Check sheet for the modelled part. Datum: model origin and axes. Units: mm. Coordinates: 2 decimals unless noted, no trailing zeros. Loops run counter-clockwise (first coordinate to the right, second up) from the corner with the lowest first, then second, coordinate; pieces in that order, holes last. Notation, with made-up numbers: M 71.5,57.25 L 95.5,57.25 A30 ccw 95.5,86.25 Z; hole C 62.25,54 d8. An arc over 180 degrees is marked long. Write each question's results on one line, items separated by ' | '. Start each with the question number.
from build123d import *

# Parameters (mm, degrees)
SKETCH1_R           = 16.1655
BOSS_EXTRUDE1_DEPTH = 13.5
FILLET1_R           = 1
SKETCH2_R           = 12.5
SKETCH2_R_2         = 11
BOSS_EXTRUDE2_DEPTH = 1
FILLET4_R           = 0.707


with BuildPart() as part:
    # Sketch1 → Boss-Extrude1 (new body)
    with BuildSketch(Plane(origin=(0, 0, 0), x_dir=(1, 0, 0), z_dir=(0, 1, 0))):
        Circle(SKETCH1_R)
    extrude(amount=BOSS_EXTRUDE1_DEPTH)

    # Fillet1
    fillet1_edges = [part.edges().sort_by_distance(p)[0] for p in [
        (-16.1655, 0, 0),
        (-16.1655, 13.5, 0),
    ]]
    fillet(fillet1_edges, radius=FILLET1_R)

    # Sketch2 → Boss-Extrude2 (add)
    with BuildSketch(Plane(origin=(0, 13.5, 0), x_dir=(1, 0, 0), z_dir=(0, 1, 0))):
        Circle(SKETCH2_R)
        Circle(SKETCH2_R_2, mode=Mode.SUBTRACT)
    extrude(amount=BOSS_EXTRUDE2_DEPTH)

    # Fillet4
    fillet4_edges = [part.edges().sort_by_distance(p)[0] for p in [
        (-12.5, 14.5, 0),
        (-11, 14.5, 0),
    ]]
    fillet(fillet4_edges, radius=FILLET4_R)


solid = part.part
Item 1: Release check for a two-part mould opening along X. For faces 1 (the face through (15.419, 6.67, -4.856)), 2 (the face through (0, 0, 0)), 3 (the face through (0, 13.5, 0)) record: +X half, -X half, draft (parallel to the pull), parting line (faces both ways), or undercut.
Item 2: Section check B-B (z = 0). Record the cut outline in (x, y).
Item 3: Depth check by flat-ended pin: P1, Ø10, axis at x = -9, z = -7, coming from the -Y side; P2, Ø2, axis at y = 11, z = -7.5, coming from the +X side; P3, Ø2, axis at x = -2.5, z = 8.5, coming from the +Y side; P4, Ø2, axis at y = 11.5, z = 11.5, coming from the +X side. Enter the tip coordinate at first touch or a pass-through.
Item 4: Thickness scan on line 1 (X direction, y = 13.75, z = 0); line 2 (Y direction, x = 6, z = -6). Record the ranges inside material, lowest first.
Item 5: Section check A-A (x = 0). Record the cut outline in (y, z).
Item 6: Section check C-C (y = 2.5). Record the cut outline in (x, z), plus the area to 3 significant figures.
Computed values:
1) face 1: parting line | face 2: draft | face 3: undercut
2) outline: M -16.17,1 A1 ccw -15.17,0 L 15.17,0 A1 ccw 16.17,1 L 16.17,12.5 A1 ccw 15.17,13.5 L 12.5,13.5 L 12.5,13.79 A0.71 ccw 11.79,14.5 L 11.71,14.5 A0.71 ccw 11,13.79 L 11,13.5 L -11,13.5 L -11,13.79 A0.71 ccw -11.71,14.5 L -11.79,14.5 A0.71 ccw -12.5,13.79 L -12.5,13.5 L -15.17,13.5 A1 ccw -16.17,12.5 Z
3) P1: stops at y = 0 | P2: stops at x = 14.8 | P3: stops at y = 13.5 | P4: stops at x = 12.29
4) line 1: x = -12.5 to -11, 11 to 12.5 | line 2: y = 0 to 13.5
5) outline: M 0,-15.17 A1 ccw 1,-16.17 L 12.5,-16.17 A1 ccw 13.5,-15.17 L 13.5,-12.5 L 13.79,-12.5 A0.71 ccw 14.5,-11.79 L 14.5,-11.71 A0.71 ccw 13.79,-11 L 13.5,-11 L 13.5,11 L 13.79,11 A0.71 ccw 14.5,11.71 L 14.5,11.79 A0.71 ccw 13.79,12.5 L 13.5,12.5 L 13.5,15.17 A1 ccw 12.5,16.17 L 1,16.17 A1 ccw 0,15.17 Z
6) outline: C 0,0 d32.33 | area: 821 mm²
